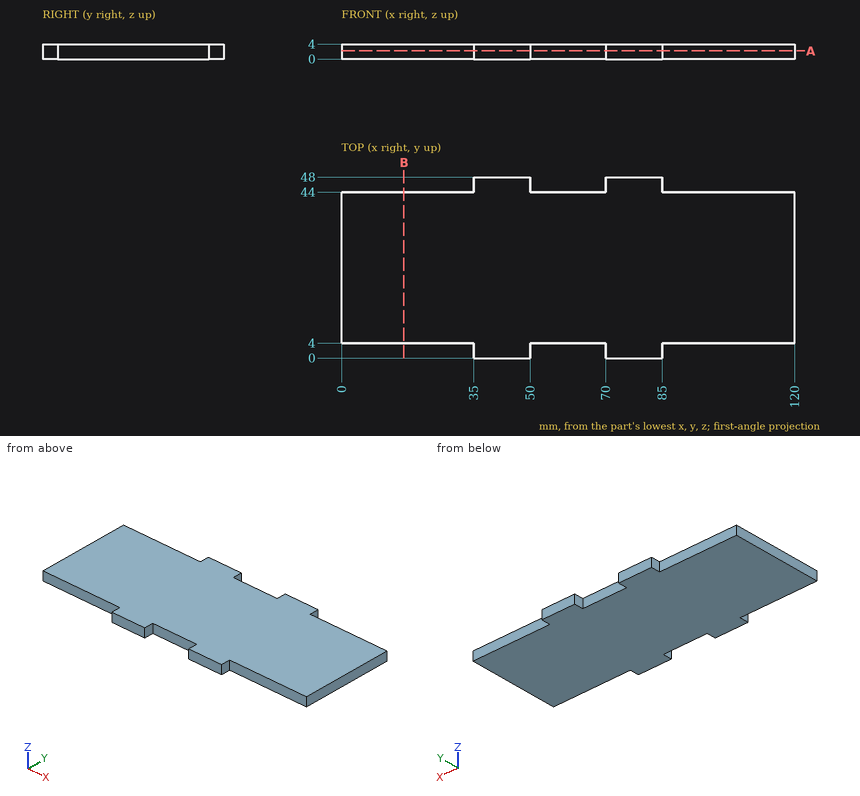
Check sheet for the drawn part. Datum: minimum x, y, z corner. Units: mm. Give positions to 0.01 mm unless a question says otherwise; leave off trailing zeros. Order: outer loops, then holes, each group sorted by start corner. A loop starts at its lowest first (then second) coordinate and runs counter-clockwise, first axis right, second up. Notation, with made-up numbers: (77.5, -18.75) - (100.5, -18.75) arc R15 ccw to (100.5, -2.75) - close; hole circle Ø1 at (45.25, 33.25). An arc over 180 degrees is marked (long way). Answer in a Markdown table with one row per item. Add a question column.
Q1. Cross-section at B-B, the plane x = 16.5. Enter the section's corners in (y, z), then the cut area to 3 significant figures.
Q2. Gauge pin test, flat ends, axial feed: pin 1 (2 mm diameter, centred on x = 59.5, z = 2, fed in from -Y); pin 2 (2 mm diameter, centred on x = 11, z = 2.5, fed in from +Y); pin 3 (2 mm diameter, centred on y = 46.5, z = 3, fed in from -X). Record the tip position at first contact, or that the pin passes through.
Q3. Cross-section at A-A, the plane z = 2.2. Enter the section's corners in (x, y), then the cut area to 3 significant figures.
Q4. Material ranges on probe 1 along Y at (x, z) = (90.5, 3), recorded low to high. Write a range as from..to.
Check values:
| question | item | result |
|---|---|---|
| 1 | outline | (4, 0) - (44, 0) - (44, 4) - (4, 4) - close |
| 1 | area | 160 mm^2 |
| 2 | pin 1 | stops at y = 4 |
| 2 | pin 2 | stops at y = 44 |
| 2 | pin 3 | stops at x = 35 |
| 3 | outline | (0, 4) - (35, 4) - (35, 0) - (50, 0) - (50, 4) - (70, 4) - (70, 0) - (85, 0) - (85, 4) - (120, 4) - (120, 44) - (85, 44) - (85, 48) - (70, 48) - (70, 44) - (50, 44) - (50, 48) - (35, 48) - (35, 44) - (0, 44) - close |
| 3 | area | 5,040 mm^2 |
| 4 | probe 1 | y = 4..44 |
